from build123d import *

# Parameters (mm, degrees)
BOSS_EXTRUDE1_DEPTH  = 100
M3_CLEARANCE_HOLE1_D = 3.4
SKETCH4_R            = 3.25
CUT_EXTRUDE1_DEPTH   = 108.964114408


with BuildPart() as part:
    # Sketch1 → Boss-Extrude1 (new body)
    with BuildSketch(Plane(origin=(0, 0, 0), x_dir=(0, 0, -1), z_dir=(1, 0, 0))):
        Polygon((0, 0), (0, 30), (-5, 30), (-9.312388631, 5.54322876), (-30, 0), align=None)
    extrude(amount=BOSS_EXTRUDE1_DEPTH)

    # M3 Clearance Hole1 (through all)
    with Locations(Plane(origin=(0, 0, 0), x_dir=(-1, 0, 0), z_dir=(0, 0, -1))):
        with Locations((-25, 15), (-75, 15)):
            Hole(M3_CLEARANCE_HOLE1_D / 2)

    # Sketch4 → Cut-Extrude1 (cut, through all)
    with BuildSketch(Plane(origin=(0, 0, 2.5), x_dir=(-1, 0, 0), z_dir=(0, 0, -1))):
        with Locations((-75, 15)):
            Circle(SKETCH4_R)
        with Locations((-25, 15)):
            Circle(SKETCH4_R)
    extrude(amount=-CUT_EXTRUDE1_DEPTH, mode=Mode.SUBTRACT)


solid = part.part
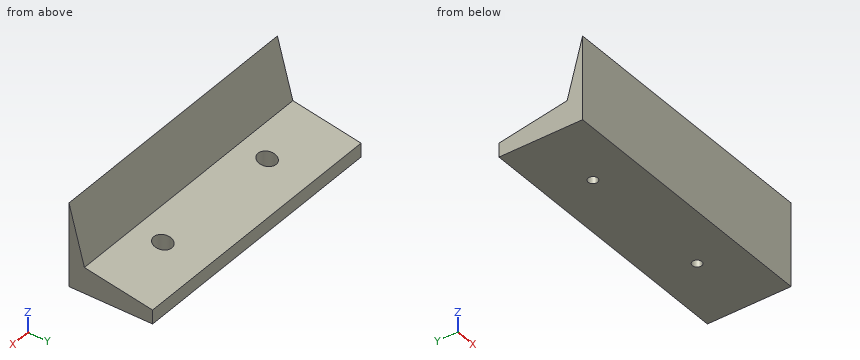
The model under review builds one solid part; all positions refer to its coordinate system, in mm. Give positions to 0.01 mm unless a question says otherwise; leave off trailing zeros. Order: outer loops, then holes, each group sorted by start corner. A loop starts at its lowest first (then second) coordinate and runs counter-clockwise, first axis right, second up. Notation, with made-up numbers: (0, 45) -> (32, 45) arc R25 ccw to (32, 70) -> close; hole circle Ø6 at (14, -23). An arc over 180 degrees is marked (long way). Write item = value, one per line. Start each with the question number.
(1) For pin 1 Ø1.5 at (x, y) = (53, 19) entering from -Z; pin 2 Ø5 at (x, y) = (74.5, 14) entering from +Z; pin 3 Ø3 at (x, y) = (25, 16.5) entering from +Z; pin 4 Ø3 at (x, y) = (25, 15) entering from +Z, all flat-tipped, find the tip position at first contact; note any pin that passes through.
(2) Take a section at B-B (y = 15). Write out the cut boundary in (x, z), plus the area to 3 significant figures.
(3) For L1, parallel to X at y = 15, z = 6.65; L2, parallel to Y at x = 75, z = 1.05; L3, parallel to Z at x = 48, y = 12.25, list the stretches that pass through material, from the lowest coordinate up. Write a range as from..to.
(4) Take a section at D-D (y = 8). Write out the cut boundary in (x, z), plus the area to 3 significant figures.
(5) Take a section at A-A (x = 75). Write out the cut boundary in (y, z).
(6) Take a section at C-C (x = 64.5). Write out the cut boundary in (y, z).
Returned:
q1.pin_1 = 0
q1.pin_2 = 8.26
q1.pin_3 = 2.5
q1.pin_4 = through
q2.outline = (0, 0) -> (23.3, 0) -> (23.3, 2.5) -> (21.75, 2.5) -> (21.75, 7.64) -> (0, 7.64) -> close; (26.7, 0) -> (73.3, 0) -> (73.3, 2.5) -> (71.75, 2.5) -> (71.75, 7.64) -> (28.25, 7.64) -> (28.25, 2.5) -> (26.7, 2.5) -> close; (76.7, 0) -> (100, 0) -> (100, 7.64) -> (78.25, 7.64) -> (78.25, 2.5) -> (76.7, 2.5) -> close
q2.area = 681 mm²
q3.L1 = 0..21.75, 28.25..71.75, 78.25..100
q3.L2 = 0..13.3, 16.7..30
q3.L3 = 0..8.13
q4.outline = (0, 0) -> (100, 0) -> (100, 8.88) -> (0, 8.88) -> close
q4.area = 888 mm²
q5.outline = (0, 0) -> (13.3, 0) -> (13.3, 2.5) -> (11.75, 2.5) -> (11.75, 8.22) -> (5.54, 9.31) -> (0, 30) -> close; (16.7, 0) -> (30, 0) -> (30, 5) -> (18.25, 7.07) -> (18.25, 2.5) -> (16.7, 2.5) -> close
q6.outline = (0, 0) -> (30, 0) -> (30, 5) -> (5.54, 9.31) -> (0, 30) -> close
